Work out the finished part from the listing and answer in its coordinate system (mm). A direction names the side the tool comes from. Give positions to 0.01 mm unless a question says otherwise; leave off trailing zeros. Order: outer loops, then holes, each group sorted by start corner. A loop starts at its lowest first (then second) coordinate and runs counter-clockwise, first axis right, second up. Notation, with made-up numbers: (-5.5, 33.5) - (-1.5, 33.5) arc R27 cw to (-1.5, 60.5) - close; hole circle Ø5 at (76, 16). An arc over 180 degrees is marked (long way). Put each result on its own line as item: value.
```python
from build123d import *

# Parameters (mm, degrees)
F0_W     = 31.75
F0_H     = 25.4
F1_DEPTH = 3.175
F2_W     = 3.4544
F2_H     = 25.4
F3_DEPTH = 7.62
F4_R     = 1.27
F5_R     = 1.905
F6_DEPTH = 3.175


with BuildPart() as f1:
    # F0 (on Top) → F1 (new body)
    with BuildSketch(Plane.XY):
        Rectangle(F0_W, F0_H)
    extrude(amount=F1_DEPTH)

    # F2 (on face) → F3 (join)
    with BuildSketch(Plane.XY.offset(3.175)):
        with Locations((-3.3528, 0)):
            Rectangle(F2_W, F2_H)
        with Locations((3.3528, 0)):
            Rectangle(F2_W, F2_H)
    extrude(amount=F3_DEPTH)

    # F4
    f4_edges = [f1.edges().sort_by_distance(p)[0] for p in [
        (-1.6256, 0, 10.795),
        (-5.08, 0, 10.795),
        (1.6256, 0, 10.795),
        (5.08, 0, 10.795),
        (1.6256, 12.7, 6.985),
        (-1.6256, 12.7, 6.985),
        (1.6256, -12.7, 6.985),
        (-1.6256, -12.7, 6.985),
    ]]
    fillet(f4_edges, radius=F4_R)

    # F5 (on face) → F6 (cut, through all)
    with BuildSketch(Plane.XY.offset(3.175)):
        with Locations((-10.16, 6.35)):
            Circle(F5_R)
        with Locations((10.16, -6.35)):
            Circle(F5_R)
    extrude(amount=-F6_DEPTH, mode=Mode.SUBTRACT)


solid = f1.part
```
(1) Section D-D, the plane y = -1.5 is taken. Write down the section's boundary in (x, z) (3 decimals), then the cut area to 3 significant figures.
Geometry check:
outline: (-15.875, 0) - (15.875, 0) - (15.875, 3.175) - (5.08, 3.175) - (5.08, 9.525) arc R1.27 ccw to (3.81, 10.795) - (2.896, 10.795) arc R1.27 ccw to (1.626, 9.525) - (1.626, 3.175) - (-1.626, 3.175) - (-1.626, 9.525) arc R1.27 ccw to (-2.896, 10.795) - (-3.81, 10.795) arc R1.27 ccw to (-5.08, 9.525) - (-5.08, 3.175) - (-15.875, 3.175) - close
area: 152 mm²
(2) Determine the mould class of faces 4 (the face through (15.875, 0, 2)), 5 (the face through (-3.4, 0.2, 10.795)), 6 (the face through (1.988, 0.178, 10.413)), 7 (the face through (-15.875, 0, 2)) for opening direction X: pulls with the +X half, pulls with the -X half, needs draft (parallel to the pull), parting line crosses it, or undercut.
Geometry check:
face 4: pulls with the +X half
face 5: needs draft
face 6: undercut
face 7: pulls with the -X half
(3) Straight lines are drawn through the part: line 1 (Y direction, x = 10.16, z = 2.2) (3 decimals); line 2 (X direction, y = -2, z = 6.5); line 3 (Y direction, x = -10.16, z = 0.95) (3 decimals). For each, find the intervals that lie inside material, in ascending order.
Geometry check:
line 1: y = -12.7 to -8.255, -4.445 to 12.7
line 2: x = -5.08 to -1.63, 1.63 to 5.08
line 3: y = -12.7 to 4.445, 8.255 to 12.7
(4) A tool of negligible diameter and unlimited length cuts with its end or side. For faces 1 (the face through (-11, 0, 3.175)), 2 (the face through (5.08, 0, 6)), 3 (the face through (-1.988, 0.178, 10.413)), from which of +Z, -Z, +X, -X, +Y, -Y can it reach the whole face along a straight path? Write none if from no direction.
Geometry check:
face 1: +Z, -X, +Y, -Y
face 2: +Z, +X, +Y, -Y
face 3: +Z, +Y, -Y
(5) Section B-B, the plane y = -6.35 is taken. Write down the section's boundary in (x, z) (3 decimals).
Geometry check:
outline: (-15.875, 0) - (8.255, 0) - (8.255, 3.175) - (5.08, 3.175) - (5.08, 9.525) arc R1.27 ccw to (3.81, 10.795) - (2.896, 10.795) arc R1.27 ccw to (1.626, 9.525) - (1.626, 3.175) - (-1.626, 3.175) - (-1.626, 9.525) arc R1.27 ccw to (-2.896, 10.795) - (-3.81, 10.795) arc R1.27 ccw to (-5.08, 9.525) - (-5.08, 3.175) - (-15.875, 3.175) - close; (12.065, 0) - (15.875, 0) - (15.875, 3.175) - (12.065, 3.175) - close
(6) Section C-C, the plane z = 7.25 is taken. Write down the section's boundary in (x, y).
Geometry check:
outline: (-5.08, -12.7) - (-2.9, -12.7) arc R1.27 ccw to (-1.63, -11.43) - (-1.63, 11.43) arc R1.27 ccw to (-2.9, 12.7) - (-5.08, 12.7) - close; (1.63, -11.43) arc R1.27 ccw to (2.9, -12.7) - (5.08, -12.7) - (5.08, 12.7) - (2.9, 12.7) arc R1.27 ccw to (1.63, 11.43) - close
(7) Given pin 1 (12 mm diameter, centred on x = 10, y = 2.5, fed in from +Z); pin 2 (3 mm diameter, centred on y = -9.5, z = 6, fed in from +X); pin 3 (1.5 mm diameter, centred on y = -9.5, z = 7.5, fed in from -X); pin 4 (2.5 mm diameter, centred on x = -10.16, y = 6.35, fed in from -Z), each flat-ended and moving along its own axis, determine where each tip first touches the part or whether it passes through.
Geometry check:
pin 1: stops at z = 10.78
pin 2: stops at x = 5.08
pin 3: stops at x = -5.08
pin 4: passes through
(8) Section A-A, the plane x = 10.16 is taken. Write down the section's boundary in (y, z) (3 decimals), then the cut area to 3 significant figures.
Geometry check:
outline: (-12.7, 0) - (-8.255, 0) - (-8.255, 3.175) - (-12.7, 3.175) - close; (-4.445, 0) - (12.7, 0) - (12.7, 3.175) - (-4.445, 3.175) - close
area: 68.5 mm²
